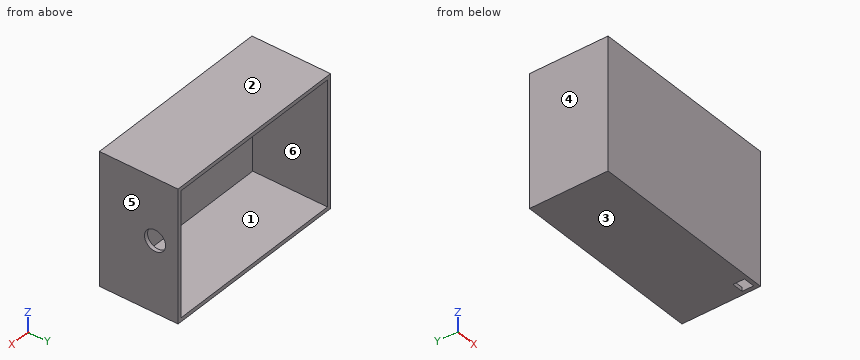
```python
from build123d import *

# Parameters (mm, degrees)
SKETCH1_W           = 100
SKETCH1_H           = 69
BOSS_EXTRUDE1_DEPTH = 41
SKETCH3_W           = 96
SKETCH3_H           = 65
CUT_EXTRUDE2_DEPTH  = 39
SKETCH4_W           = 6
SKETCH4_H           = 6
CUT_EXTRUDE3_DEPTH  = 2
SKETCH1_4_W         = 100
SKETCH1_4_H         = 69
BOSS_EXTRUDE2_DEPTH = 2
SKETCH6_R           = 5.5
CUT_EXTRUDE4_DEPTH  = 2


with BuildPart() as part:
    # Sketch1 → Boss-Extrude1 (new body)
    with BuildSketch(Plane(origin=(0, 0, 0), x_dir=(1, 0, 0), z_dir=(0, 1, 0))):
        Rectangle(SKETCH1_W, SKETCH1_H)
    extrude(amount=BOSS_EXTRUDE1_DEPTH)

    # Sketch3 → Cut-Extrude2 (cut)
    with BuildSketch(Plane(origin=(0, 41, 0), x_dir=(1, 0, 0), z_dir=(0, 1, 0))):
        Rectangle(SKETCH3_W, SKETCH3_H)
    extrude(amount=-CUT_EXTRUDE2_DEPTH, mode=Mode.SUBTRACT)

    # Sketch4 → Cut-Extrude3 (cut)
    with BuildSketch(Plane(origin=(0, 0, -34.5), x_dir=(-1, 0, 0), z_dir=(0, 0, -1))):
        with Locations((-45, 5)):
            Rectangle(SKETCH4_W, SKETCH4_H)
    extrude(amount=-CUT_EXTRUDE3_DEPTH, mode=Mode.SUBTRACT)

    # Sketch1<4> → Boss-Extrude2 (add)
    with BuildSketch(Plane(origin=(0, 0, 0), x_dir=(1, 0, 0), z_dir=(0, 1, 0))):
        Rectangle(SKETCH1_4_W, SKETCH1_4_H)
    extrude(amount=BOSS_EXTRUDE2_DEPTH)

    # Sketch6 → Cut-Extrude4 (cut)
    with BuildSketch(Plane(origin=(50, 0, 0), x_dir=(0, 0, -1), z_dir=(1, 0, 0))):
        with Locations((-2.5, 29)):
            Circle(SKETCH6_R)
    extrude(amount=-CUT_EXTRUDE4_DEPTH, mode=Mode.SUBTRACT)


solid = part.part
```
The model under review builds one solid part; all positions refer to its coordinate system, in mm. Face numbers are marked on the shaded views. A direction names the side the tool comes from. Round coordinates to 2 decimals unless told otherwise and drop trailing zeros. Write each loop counter-clockwise with the first axis right and the second up, starting at its lowest first coordinate (ties: lowest second). Pieces come first, ordered by that corner, then holes. Notation, with made-up numbers: (-28, -33) - (0, -33) arc R30 ccw to (0, -1) - close; hole circle Ø10 at (72, 74). An arc over 180 degrees is marked (long way). Answer as CSV lines item,"result". Start each with the question number.
(1) For the marked faces 5 and 6, list the 3-axis set-ups (+Z, -Z, +X, -X, +Y, -Y) from which the entire face can be reached by the end or side of a thin tool; tool diameter is ignored.
(2) We need section C-C on y = 29. State the section outline as (x, z) points, plus the area to 3 significant figures.
(3) We need section A-A on z = 2.5. State the section outline as (x, y) points.
(4) To check wall thickness, follow line 1 (X direction, y = 18, z = -28.5); line 2 (Z direction, x = -21, y = 36.5); line 3 (Y direction, x = 49.6, z = 2.5). State the ranges of each line that lie inside material, in increasing order.
(5) We need section D-D on x = 39. State the section outline as (y, z) points, plus the area to 3 significant figures.
(6) We need section B-B on z = -18. State the section outline as (x, y) points.
(7) For pin 1 Ø2 at (x, z) = (-8.5, -12.5) entering from +Y, flat-tipped, find the tip position at first contact; note if it passes through.
(8) Draft analysis for pull direction Z (two halves, no side actions). For the marked faces 1, 2, 3 and 4, state which applies: pulls with the +Z half, pulls with the -Z half, needs draft (parallel to the pull), parting line crosses it, or undercut.
Worked answers:
1,face 5,"+Z, -Z, +X, +Y, -Y"
1,face 6,"+Y"
2,outline,"(-50, -34.5) - (50, -34.5) - (50, -3) - (48, -3) - (48, -32.5) - (-48, -32.5) - (-48, 32.5) - (48, 32.5) - (48, 8) - (50, 8) - (50, 34.5) - (-50, 34.5) - close"
2,area,"638 mm²"
3,outline,"(-50, 0) - (50, 0) - (50, 23.5) - (48, 23.5) - (48, 2) - (-48, 2) - (-48, 41) - (-50, 41) - close; (48, 34.5) - (50, 34.5) - (50, 41) - (48, 41) - close"
4,line 1,"-50 to -48, 48 to 50"
4,line 2,"-34.5 to -32.5, 32.5 to 34.5"
4,line 3,"0 to 23.5, 34.5 to 41"
5,outline,"(0, -34.5) - (41, -34.5) - (41, -32.5) - (2, -32.5) - (2, 32.5) - (41, 32.5) - (41, 34.5) - (0, 34.5) - close"
5,area,"294 mm²"
6,outline,"(-50, 0) - (50, 0) - (50, 41) - (48, 41) - (48, 2) - (-48, 2) - (-48, 41) - (-50, 41) - close"
7,pin 1,"y = 2"
8,face 1,"undercut"
8,face 2,"pulls with the +Z half"
8,face 3,"pulls with the -Z half"
8,face 4,"needs draft"
